The drawing under review shows one solid part. Ordinate dimensions are in mm from its lowest x, y, z. Give positions to 0.01 mm unless a question says otherwise; leave off trailing zeros. Loops run counter-clockwise (first coordinate to the right, second up) from the corner with the lowest first, then second, coordinate; pieces in that order, holes last.
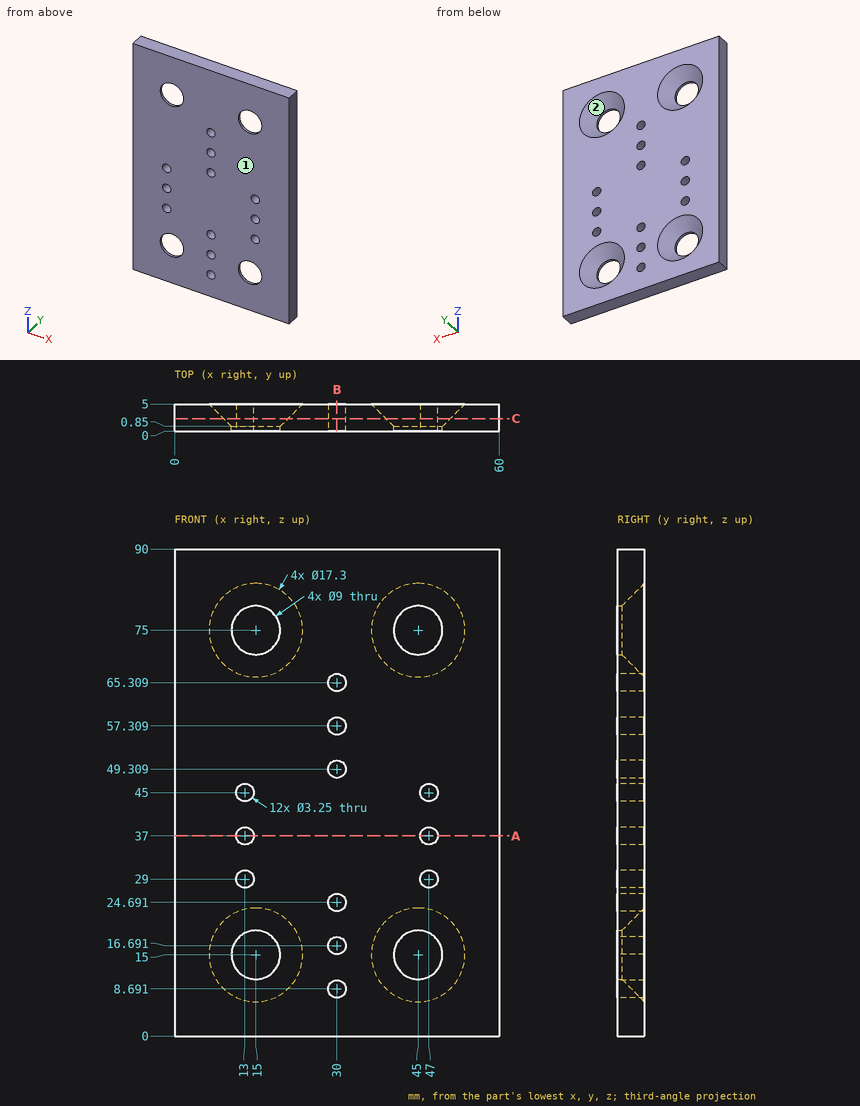
Item 1: Take a section at B-B on x = 30. Give the boundary of the cut face in (y, z), and give its area (4 significant figures).
Answer:
outline: (0, 0) - (5, 0) - (5, 7.07) - (0, 7.07) - close; (0, 10.32) - (5, 10.32) - (5, 15.07) - (0, 15.07) - close; (0, 18.32) - (5, 18.32) - (5, 23.07) - (0, 23.07) - close; (0, 26.32) - (5, 26.32) - (5, 47.68) - (0, 47.68) - close; (0, 50.93) - (5, 50.93) - (5, 55.68) - (0, 55.68) - close; (0, 58.93) - (5, 58.93) - (5, 63.68) - (0, 63.68) - close; (0, 66.93) - (5, 66.93) - (5, 90) - (0, 90) - close
area: 352.5 mm2
Item 2: Take a section at A-A on z = 37. Give the boundary of the cut face in (x, y) (3 decimals).
Answer:
outline: (0, 0) - (11.375, 0) - (11.375, 5) - (0, 5) - close; (14.625, 0) - (45.375, 0) - (45.375, 5) - (14.625, 5) - close; (48.625, 0) - (60, 0) - (60, 5) - (48.625, 5) - close
Item 3: The part is to be moulded in two halves that separate along X. For the marked faces 1 and 2, say which applies: released by +X, released by -X, zero draft, split by the parting line, or undercut.
Answer:
face 1: zero draft
face 2: undercut
Item 4: Take a section at C-C on y = 2.3. State how many separate pieces and enclosed holes the cut face has, and give its area (3 significant figures).
Answer:
separate pieces: 1
enclosed holes: 16
area: 4,860 mm2
Item 5: For L1, parallel to Z at x = 15, y = 0.3; L2, parallel to X at y = 0.4, z = 15; L3, parallel to X at y = 1.2, z = 37 (3 decimals), list the stretches that pass through material, from the lowest coordinate up.
Answer:
L1: z = 0 to 10.5, 19.5 to 70.5, 79.5 to 90
L2: x = 0 to 10.5, 19.5 to 40.5, 49.5 to 60
L3: x = 0 to 11.375, 14.625 to 45.375, 48.625 to 60
